The model under review builds one solid part; all positions refer to its coordinate system, in mm. A direction names the side the tool comes from. Round coordinates to 2 decimals unless told otherwise and drop trailing zeros. Write each loop counter-clockwise with the first axis right and the second up, starting at its lowest first coordinate (ties: lowest second). Pieces come first, ordered by that corner, then holes. Notation, with made-up numbers: M 48.5,-9.75 L 55.5,-9.75 A11 ccw 55.5,9.25 Z; hole C 27,32 d7. An arc over 180 degrees is marked long. Write item = value, one per line. Start each with the question number.
Item 1: Take a section at D-D, the plane z = 2. Give the boundary of the cut face in (x, y), plus the area to 3 significant figures.
Item 2: The part is to be moulded in two halves that separate along X. For faces 1 (the flat face through (2, 21, -2)), 2 (the cylindrical face through (-0.867, 10.353, 3.905)), 3 (the cylindrical face through (-1.5, 10.75, -0.07)), say which applies: +X half, -X half, draft (parallel to the pull), parting line (faces both ways), or undercut.
Item 3: For pin 1 Ø2 at (y, z) = (24, 1) entering from -X; pin 2 Ø1 at (x, y) = (1.5, 18) entering from -Z, all flat-tipped, find the tip position at first contact; note any pin that passes through.
Item 4: Tool access review of faces 4 (the flat face through (0, 28.5, 2)), 5 (the flat face through (2, 0, -2)), 6 (the cylindrical face through (-0.54, 24.7, 2.44)): name each direction out of +Z, -Z, +X, -X, +Y, -Y from which nothing blocks a thin tool from reaching the whole face with its end or side.
Item 5: Take a section at C-C, the plane y = -2.5. Give the boundary of the cut face in (x, z).
Item 6: Take a section at A-A, the plane x = 0. Give the boundary of the cut face in (y, z), plus the area to 3 significant figures.
Item 7: To check wall thickness, follow line 1 along X through (y, z) = (4.5, 0); line 2 along Y through (x, z) = (-2.5, 1.5). State the ranges of each line that lie inside material, in increasing order.
Item 8: Take a section at B-B, the plane z = 0. Give the boundary of the cut face in (x, y).
from build123d import *

# Parameters (mm, degrees)
SKETCH1_R           = 4
SKETCH1_R_2         = 1.25
BOSS_EXTRUDE1_DEPTH = 21
SKETCH2_R           = 2.5
BOSS_EXTRUDE2_DEPTH = 7.5
SKETCH3_R           = 2.5
BOSS_EXTRUDE3_DEPTH = 7.5
SKETCH4_R           = 1.5
CUT_EXTRUDE1_DEPTH  = 37


with BuildPart() as part:
    # Sketch1 → Boss-Extrude1 (new body)
    with BuildSketch(Plane(origin=(0, 0, 0), x_dir=(1, 0, 0), z_dir=(0, 1, 0))):
        Circle(SKETCH1_R)
        Circle(SKETCH1_R_2, mode=Mode.SUBTRACT)
    extrude(amount=BOSS_EXTRUDE1_DEPTH)

    # Sketch2 → Boss-Extrude2 (add)
    with BuildSketch(Plane.XZ):
        Circle(SKETCH2_R)
    extrude(amount=BOSS_EXTRUDE2_DEPTH)

    # Sketch3 → Boss-Extrude3 (add)
    with BuildSketch(Plane(origin=(0, 21, 0), x_dir=(1, 0, 0), z_dir=(0, 1, 0))):
        Circle(SKETCH3_R)
    extrude(amount=BOSS_EXTRUDE3_DEPTH)

    # Sketch4 → Cut-Extrude1 (cut, through all)
    with BuildSketch(Plane(origin=(0, 28.5, 0), x_dir=(1, 0, 0), z_dir=(0, 1, 0))):
        Circle(SKETCH4_R)
    extrude(amount=-CUT_EXTRUDE1_DEPTH, mode=Mode.SUBTRACT)


solid = part.part
Response values:
q1.outline = M -3.46,0 L -1.5,0 L -1.5,-7.5 L 1.5,-7.5 L 1.5,0 L 3.46,0 L 3.46,21 L 1.5,21 L 1.5,28.5 L -1.5,28.5 L -1.5,21 L -3.46,21 Z
q1.area = 190 mm2
q2.face_1 = draft
q2.face_2 = parting line
q2.face_3 = undercut
q3.pin_1 = -2.5
q3.pin_2 = -3.87
q4.face_4 = +Z, -Z, +X, -X, +Y
q4.face_5 = -Y
q4.face_6 = +Y
q5.outline = C 0,0 d5; hole C 0,0 d3
q6.outline = M -7.5,-2.5 L 0,-2.5 L 0,-4 L 21,-4 L 21,-2.5 L 28.5,-2.5 L 28.5,-1.5 L -7.5,-1.5 Z; M -7.5,1.5 L 28.5,1.5 L 28.5,2.5 L 21,2.5 L 21,4 L 0,4 L 0,2.5 L -7.5,2.5 Z
q6.area = 135 mm2
q7.line_1 = -4 to -1.5, 1.5 to 4
q7.line_2 = 0 to 21
q8.outline = M -4,0 L -2.5,0 L -2.5,-7.5 L -1.5,-7.5 L -1.5,28.5 L -2.5,28.5 L -2.5,21 L -4,21 Z; M 1.5,-7.5 L 2.5,-7.5 L 2.5,0 L 4,0 L 4,21 L 2.5,21 L 2.5,28.5 L 1.5,28.5 Z
